Job drawing, mm, ordinate dimensions from the low corner. One solid piece. Coordinates: 2 decimals unless noted, no trailing zeros. Write each loop counter-clockwise with the first axis right and the second up, starting at its lowest first coordinate (ties: lowest second). Pieces come first, ordered by that corner, then holes. Notation, with made-up numbers: (12, 87) - (44, 87) arc R5 ccw to (44, 95) - close; hole circle Ø3 at (87.5, -9.75). An arc over 180 degrees is marked (long way). Use one line per item in the form item = value. Start each with the question number.
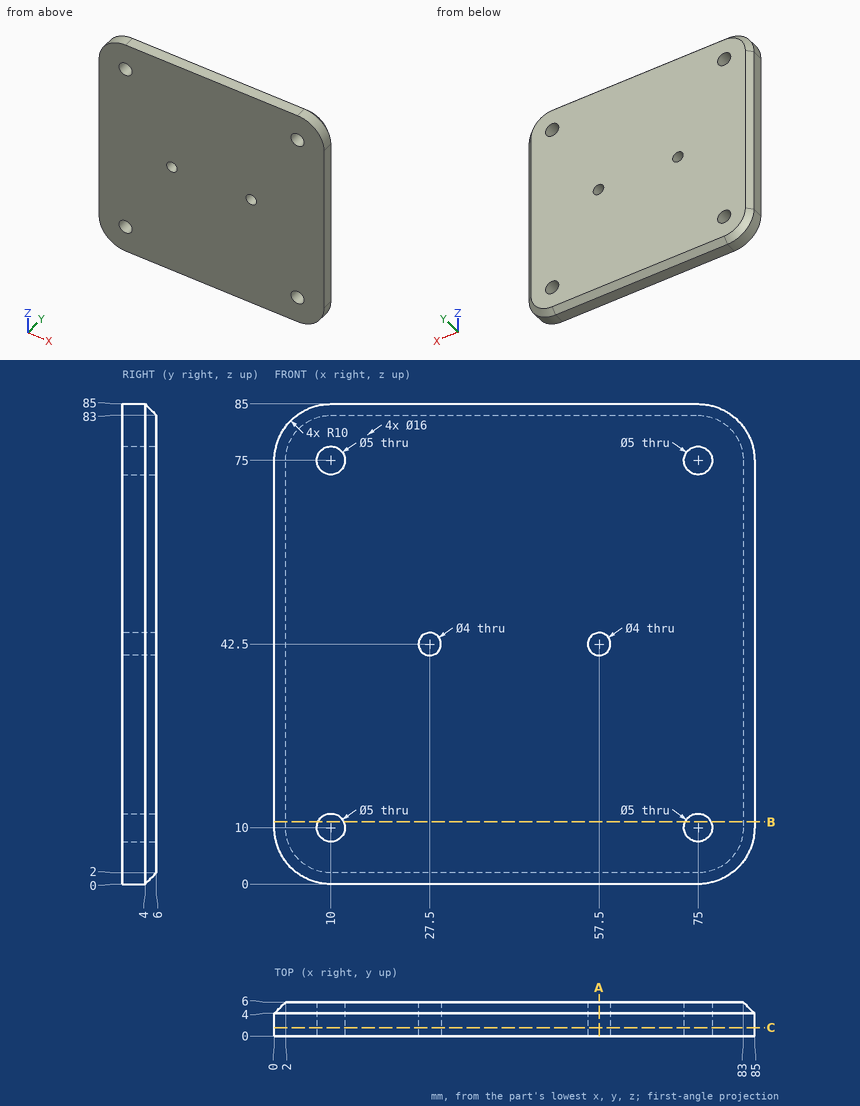
Q1. Slice it at B-B (z = 11). List the corners of the cut face in (x, y).
Q2. Slice it at C-C (y = 1.5). List the corners of the cut face in (x, z), plus the area to 3 significant figures.
Q3. Slice it at A-A (x = 57.5). List the corners of the cut face in (y, z).
Q4. Pin check, flat tip, straight feed: P1, Ø2.5, axis at x = 27.5, z = 42.5, coming from the -Y side. Stop position of the tip, or through.
Q5. Drill centre lines: probe 1 along Z at (x, y) = (75, 3.6); probe 2 along X at (y, z) = (2.5, 42.5); probe 3 along X at (y, z) = (4.3, 75). Where is each one in solid material? Low to high.
Solution:
q1.outline = (0, 0) - (7.71, 0) - (7.71, 6) - (2, 6) - (0, 4) - close; (12.29, 0) - (72.71, 0) - (72.71, 6) - (12.29, 6) - close; (77.29, 0) - (85, 0) - (85, 4) - (83, 6) - (77.29, 6) - close
q2.outline = (0, 10) arc R10 ccw to (10, 0) - (75, 0) arc R10 ccw to (85, 10) - (85, 75) arc R10 ccw to (75, 85) - (10, 85) arc R10 ccw to (0, 75) - close; hole circle Ø5 at (10, 10); hole circle Ø5 at (10, 75); hole circle Ø4 at (27.5, 42.5); hole circle Ø4 at (57.5, 42.5); hole circle Ø5 at (75, 10); hole circle Ø5 at (75, 75)
q2.area = 7,040 mm2
q3.outline = (0, 0) - (4, 0) - (6, 2) - (6, 40.5) - (0, 40.5) - close; (0, 44.5) - (6, 44.5) - (6, 83) - (4, 85) - (0, 85) - close
q4.P1 = through
q5.probe_1 = 0 to 7.5, 12.5 to 72.5, 77.5 to 85
q5.probe_2 = 0 to 25.5, 29.5 to 55.5, 59.5 to 85
q5.probe_3 = 0.3 to 7.5, 12.5 to 72.5, 77.5 to 84.7
